Autodesk Inventor part; units mm, degrees
ref_plane "YZ Plane" through (0, 0, 0) normal (1, 0, 0) x (0, 1, 0)
ref_plane "XY Plane" through (0, 0, 0) normal (0, 0, 1) x (1, 0, 0)
sketch "Sketch1" plane through (0, 0, 0) normal (0, 1, 0) x (-1, 0, 0)
  circle A0 centre (0, 0) radius 32
  circle A1 centre (0, 0) radius 33
  dimension "d0" = 64
  dimension "d1" = 0
  dimension "d2" = 0
  dimension "d3" = 66
ref_plane "Work Plane1" through (0, 30, 0) normal (0, 1, 0) x (-1, 0, 0)
sketch "Sketch2" plane through (0, 30, 0) normal (0, 1, 0) x (-1, 0, 0)
  circle A0 centre (0, 0) radius 20
  circle A1 centre (0, 0) radius 21
  dimension "d5" = 40
  dimension "d6" = 42
loft "Loft1" add profiles "Sketch2", "Sketch1" contours A0 | A1 / A0 | A1
shell "Shell2" thickness 1 removed faces 0
sketch "Sketch3" plane through (0, 0, 0) normal (0, -1, 0) x (1, 0, 0)
  circle A0 centre (0, 0) radius 31.523
extrude "Extrusion1" cut sketch "Sketch3" against normal blind 1
sketch "Sketch5" plane through (0, 29, 0) normal (0, -1, 0) x (1, 0, 0)
  line L0 (11.323, 6) -> (6.323, 6)
  line L1 (6.323, 6) -> (6.323, -6)
  line L2 (6.323, -6) -> (11.323, -6)
  line L3 (11.323, -6) -> (11.323, 6)
  circle A0 centre (0, 0) radius 20.323
  circle A1 centre (0, 0) radius 6.323
  circle A2 centre (-6.323, 0) radius 2.5
  line L4 (-16.677, 6) -> (-21.677, 6)
  line L5 (-21.677, 6) -> (-21.677, -6)
  line L6 (-21.677, -6) -> (-16.677, -6)
  line L7 (-16.677, -6) -> (-16.677, 6)
  arc A3 (-19.4171, 6) -> (-19.4171, -6) centre (0, 0) ccw
  dimension "d16" = 5
  dimension "d17" = 12
  dimension "d18" = 9
  dimension "d19" = 6
  dimension "d20" = 5
  dimension "d21" = 5
  dimension "d22" = 12
  dimension "d23" = 23
extrude "Extrusion2" add sketch "Sketch5" along normal blind 7 contours L3 L2 L1 L0 | A1 A2 | A2 A1 | A1 A2 | L4 L7 L6 A0 picked at (-17.8586, -0.6756)
sketch "Sketch6" plane through (0, 22, 0) normal (0, -1, 0) x (1, 0, 0)
  arc A0 (-5.8287, 2.4507) -> (-5.8287, -2.4507) centre (-6.323, 0) ccw
  circle A1 centre (0, 0) radius 6.323
  circle A2 centre (-6.323, 0) radius 2.5
extrude "Extrusion3" cut sketch "Sketch6" against normal blind 20
sketch "Sketch7" plane through (0, 22, 0) normal (0, -1, 0) x (1, 0, 0)
  circle A0 centre (8.823, 0) radius 1
  circle A1 centre (-19.177, 0) radius 1
  line L0 (11.323, -6) -> (11.323, 6)
  line L1 (11.323, 6) -> (6.323, 6)
  line L2 (-16.677, -6) -> (-16.677, 6)
  line L3 (-16.677, 6) -> (-19.4171, 6)
  point P0 (0, 0)
  dimension "d28" = 2
  dimension "d29" = 2
  dimension "d30" = 2.5
  dimension "d31" = 6
  dimension "d32" = 2.5
  dimension "d33" = 6
extrude "Extrusion4" cut sketch "Sketch7" against normal blind 20
properties part number "zaklad"
For this review, take the finished solid that the model builds, in its own axes (mm). A direction names the side the tool comes from. Coordinates: 2 decimals unless noted, no trailing zeros. Loops run counter-clockwise (first coordinate to the right, second up) from the corner with the lowest first, then second, coordinate; pieces in that order, holes last.
1. Add section B-B, the plane y = 14. Give the boundary of the cut face in (x, z).
2. For line 1 (Y direction, x = -18.5, z = 7.5); line 2 (Z direction, x = 0, y = 0.6); line 3 (X direction, y = 7, z = -9), list the stretches that pass through material, from the lowest coordinate up.
3. Insertion check: P1, Ø5.5, axis at y = 27, z = 1.5, coming from the -X side; P2, Ø2, axis at x = -18, y = 25.5, coming from the -Z side; P3, Ø2, axis at y = 26.5, z = -0.5, coming from the +X side; P4, Ø1.6, axis at x = 8.823, z = 0, coming from the +Y side. Each pin has a flat end and moves straight along its axis. Give the tip position at first contact, or say it passes through.
4. Mouldability with a two-part tool opening along Z and no side actions: class faces 1 (the cylindrical face through (6.32, 29.49, -0.24)), 2 (the conical face through (-10.65, 24.79, 20.48)), 3 (the flat face through (-17, 0, -27)) as +Z half, -Z half, draft (parallel to the pull), parting line (faces both ways), or undercut.
5. For faces 4 (the cylindrical face through (7.824, 25.944, 0.044)), 5 (the cylindrical face through (-4.104, 0.493, 31.255)), list the 3-axis set-ups (+Z, -Z, +X, -X, +Y, -Y) from which the entire face can be reached by the end or side of a thin tool; tool diameter is ignored.
6. Add section A-A, the plane x = 0. Give the boundary of the cut face in (y, z), then the cut area to 3 significant figures.
Result:
1. outline: circle Ø54.8 at (0, 0); hole circle Ø52.65 at (0, 0)
2. line 1: y = 29 to 30
2. line 2: z = -32.76 to -31.52, 31.52 to 32.76
2. line 3: x = -28.83 to -27.7, 27.7 to 28.83
3. P1: stops at x = -23.26
3. P2: stops at z = -15.34
3. P3: stops at x = 22.8
3. P4: passes through
4. face 1: undercut
4. face 2: parting line
4. face 3: draft
5. face 4: +Y, -Y
5. face 5: -Y
6. outline: (0, -33) - (30, -21) - (30, -6.32) - (29, -6.32) - (29, -20.32) - (1, -31.52) - (0, -31.52) - close; (0, 31.52) - (1, 31.52) - (29, 20.32) - (29, 6.32) - (30, 6.32) - (30, 21) - (0, 33) - close
6. area: 92.6 mm2
